from build123d import *

# Parameters (mm, degrees)
SKETCH_2_R      = 5.03
SKETCH_2_R_2    = 2
SKETCH_2_R_3    = 1.75
EXTRUDE_1_DEPTH = 4


with BuildPart() as part:
    # 草图2 → 凸台-拉伸1 (new body)
    with BuildSketch(Plane.XY):
        with BuildLine():
            Line((-56.063767215, 68), (-262.305181408, 68))
            ThreePointArc((-262.305181408, 68), (-270.328158767, 66.320257484), (-277.003482509, 61.56318343))
            Line((-277.003482509, 61.56318343), (-322.861013463, 11.867785501))
            ThreePointArc((-322.861013463, 11.867785501), (-325.076248752, -8.885759595), (-305.846688069, -17))
            Line((-305.846688069, -17), (-56.75042146, -17))
            ThreePointArc((-56.75042146, -17), (-52.936794137, -15.632088799), (-50.862067991, -12.152082213))
            Line((-50.862067991, -12.152082213), (-37.310871287, 57.108804918))
            ThreePointArc((-37.310871287, 57.108804918), (-37.686816243, 60.630138571), (-39.983089141, 63.326108914))
            ThreePointArc((-39.983089141, 63.326108914), (-47.690693329, 66.807839796), (-56.063767215, 68))
        make_face()
        with Locations((-310, 0)):
            Circle(SKETCH_2_R, mode=Mode.SUBTRACT)
        with Locations((-225, -12)):
            Circle(SKETCH_2_R_2, mode=Mode.SUBTRACT)
        with BuildLine():
            Line((-168.599525043, 31.773817383), (-178.858293522, 9.773817383))
            ThreePointArc((-178.858293522, 9.773817383), (-182.548375309, 5.566085542), (-187.921371393, 4))
            Line((-187.921371393, 4), (-260, 4))
            ThreePointArc((-260, 4), (-281, 25), (-260, 46))
            Line((-260, 46), (-177.662602913, 46))
            ThreePointArc((-177.662602913, 46), (-169.228688455, 41.372996083), (-168.599525043, 31.773817383))
        make_face(mode=Mode.SUBTRACT)
        with Locations((-165, -12)):
            Circle(SKETCH_2_R_3, mode=Mode.SUBTRACT)
        with Locations((-145, -12)):
            Circle(SKETCH_2_R_2, mode=Mode.SUBTRACT)
        with Locations((-165, -2)):
            Circle(SKETCH_2_R_3, mode=Mode.SUBTRACT)
        with Locations((-65, -12)):
            Circle(SKETCH_2_R_2, mode=Mode.SUBTRACT)
        with BuildLine():
            Line((-139.044375749, 46), (-67.670495323, 46))
            ThreePointArc((-67.670495323, 46), (-62.94456946, 43.696704578), (-61.847044732, 38.555208246))
            Line((-61.847044732, 38.555208246), (-69.290012085, 8.555208246))
            ThreePointArc((-69.290012085, 8.555208246), (-71.416758098, 5.274074137), (-75.113462676, 4))
            Line((-75.113462676, 4), (-149.303144229, 4))
            ThreePointArc((-149.303144229, 4), (-157.737058687, 8.627003917), (-158.366222099, 18.226182617))
            Line((-158.366222099, 18.226182617), (-148.10745362, 40.226182617))
            ThreePointArc((-148.10745362, 40.226182617), (-144.417371833, 44.433914458), (-139.044375749, 46))
        make_face(mode=Mode.SUBTRACT)
        with Locations((-265, 63)):
            Circle(SKETCH_2_R_2, mode=Mode.SUBTRACT)
        with Locations((-195, 63)):
            Circle(SKETCH_2_R_2, mode=Mode.SUBTRACT)
        with Locations((-125, 63)):
            Circle(SKETCH_2_R_2, mode=Mode.SUBTRACT)
        with Locations((-55, 63)):
            Circle(SKETCH_2_R_2, mode=Mode.SUBTRACT)
    extrude(amount=EXTRUDE_1_DEPTH)


solid = part.part
The model under review builds one solid part; all positions refer to its coordinate system, in mm. A direction names the side the tool comes from. Round coordinates to 2 decimals unless told otherwise and drop trailing zeros. Loops run counter-clockwise (first coordinate to the right, second up) from the corner with the lowest first, then second, coordinate; pieces in that order, holes last. Notation, with made-up numbers: (9.25, 11.25) -> (13.25, 11.25) arc R17 cw to (13.25, 31.25) -> close; hole circle Ø9 at (57, 24). An arc over 180 degrees is marked (long way). Write item = value, one per line. Start each with the question number.
Item 1: Insertion check: pin 1 (16 mm diameter, centred on x = -310, y = 0, fed in from -Z); pin 2 (2 mm diameter, centred on y = -1, z = 3, fed in from +X); pin 3 (2 mm diameter, centred on x = -230.5, z = 2, fed in from -Y); pin 4 (1.5 mm diameter, centred on y = 57, z = 1.5, fed in from +X). Each pin has a flat end and moves straight along its axis. Give the tip position at first contact, or say it passes through.
Item 2: Take a section at D-D on x = -308.5. Give the boundary of the cut face in (y, z), plus the area to 3 significant figures.
Item 3: Take a section at B-B on z = 2.05. Count the separate pieces of the cut face and the enclosed holes in it, plus the area to 3 significant figures.
Item 4: To check wall thickness, follow L1, parallel to Y at x = -165, z = 3.1; L2, parallel to Y at x = -225, z = 1.8; L3, parallel to Y at x = -117, z = 2.5. State the ranges of each line that lie inside material, in increasing order.
Item 5: Take a section at C-C on y = 21. Give the boundary of the cut face in (x, z).
Item 6: Take a section at A-A on x = -212.5. Give the boundary of the cut face in (y, z).
Item 7: Mouldability with a two-part tool opening along X and no side actions: class faces 1 (the cylindrical face through (-157.66, 8.51, 1.97)), 2 (the cylindrical face through (-52.982, -15.669, 1.972)), 3 (the flat face through (-184, -3, 4)) as released by +X, released by -X, zero draft, split by the parting line, or undercut.
Item 8: For faces 4 (the flat face through (-44.18, 21.99, 1.97)), 5 (the flat face through (-65.516, 23.765, 1.972)), list the 3-axis set-ups (+Z, -Z, +X, -X, +Y, -Y) from which the entire face can be reached by the end or side of a thin tool; tool diameter is ignored.
Result:
q1.pin_1 = 0
q1.pin_2 = -48.48
q1.pin_3 = -17
q1.pin_4 = -37.22
q2.outline = (-17.44, 0) -> (-4.8, 0) -> (-4.8, 4) -> (-17.44, 4) -> close; (4.8, 0) -> (27.43, 0) -> (27.43, 4) -> (4.8, 4) -> close
q2.area = 141 mm²
q3.separate_pieces = 1
q3.enclosed_holes = 12
q3.area = 14,100 mm²
q4.L1 = -17 to -13.75, -10.25 to -3.75, -0.25 to 68
q4.L2 = -17 to -14, -10 to 4, 46 to 68
q4.L3 = -17 to 4, 46 to 68
q5.outline = (-314.43, 0) -> (-280.62, 0) -> (-280.62, 4) -> (-314.43, 4) -> close; (-173.62, 0) -> (-157.07, 0) -> (-157.07, 4) -> (-173.62, 4) -> close; (-66.2, 0) -> (-44.38, 0) -> (-44.38, 4) -> (-66.2, 4) -> close
q6.outline = (-17, 0) -> (4, 0) -> (4, 4) -> (-17, 4) -> close; (46, 0) -> (68, 0) -> (68, 4) -> (46, 4) -> close
q7.face_1 = undercut
q7.face_2 = released by +X
q7.face_3 = zero draft
q8.face_4 = +Z, -Z, +X, -Y
q8.face_5 = +Z, -Z
